CAD build for the part. Positions are in the model's coordinates, mm. Give positions to 0.01 mm unless a question says otherwise; leave off trailing zeros. Loops run counter-clockwise (first coordinate to the right, second up) from the corner with the lowest first, then second, coordinate; pieces in that order, holes last. Notation, with made-up numbers: M 67,46 L 90,46 A32 cw 90,76 Z; hole C -0.75,3 d5. An arc over 180 degrees is marked long. Answer as CSV lines item,"result".
```python
from build123d import *

# Parameters (mm, degrees)
ESQUISSE1_W             = 233
ESQUISSE1_H             = 150
BOSS_EXTRU_1_DEPTH      = 4.2
ESQUISSE2_R             = 2.55
ENL_V_MAT_EXTRU_1_DEPTH = 145.628460094


with BuildPart() as part:
    # Esquisse1 → Boss.-Extru.1 (new body)
    with BuildSketch(Plane.XY):
        with Locations((-3.063037439, -6.267653759)):
            Rectangle(ESQUISSE1_W, ESQUISSE1_H)
    extrude(amount=BOSS_EXTRU_1_DEPTH)

    # Esquisse2 → Enlèv. mat.-Extru.1 (cut, through all)
    with BuildSketch(Plane.XY.offset(4.2)):
        with Locations((-78.063037439, -47.267653759)):
            Circle(ESQUISSE2_R)
        with Locations((-1.063037439, -47.267653759)):
            Circle(ESQUISSE2_R)
        with BuildLine():
            Line((-69.563037439, -81.267653759), (-9.563037439, -81.267653759))
            ThreePointArc((-9.563037439, -81.267653759), (-39.563037439, -51.267653759), (-69.563037439, -81.267653759))
        make_face()
    extrude(amount=-ENL_V_MAT_EXTRU_1_DEPTH, mode=Mode.SUBTRACT)


solid = part.part
```
Q1. Cut at C-C (x = -61). Write the cut outline in (y, z), and give its area (3 significant figures).
Solution:
outline,"M -60.28,0 L 68.73,0 L 68.73,4.2 L -60.28,4.2 Z"
area,"542 mm²"
Q2. Wall check: line 1 (X direction, y = -45, z = 1.15); line 2 (X direction, y = -59, z = 1.7); line 3 (X direction, y = -64, z = 1.45). Give the ranges that are in metal, low to high. Write a range as [from, to].
Solution:
line 1,"x = [-119.56, -79.23], [-76.9, -2.23], [0.1, 113.44]"
line 2,"x = [-119.56, -59.67], [-19.46, 113.44]"
line 3,"x = [-119.56, -64.1], [-15.03, 113.44]"
Q3. Cut at A-A (y = -64.5). Write the cut outline in (x, z), and give its area (3 significant figures).
Solution:
outline,"M -119.56,0 L -64.44,0 L -64.44,4.2 L -119.56,4.2 Z; M -14.69,0 L 113.44,0 L 113.44,4.2 L -14.69,4.2 Z"
area,"770 mm²"
Q4. Cut at B-B (z = 2). Write the cut outline in (x, y).
Solution:
outline,"M -119.56,-81.27 L -69.56,-81.27 A30 cw -9.56,-81.27 L 113.44,-81.27 L 113.44,68.73 L -119.56,68.73 Z; hole C -78.06,-47.27 d5.1; hole C -1.06,-47.27 d5.1"
Q5. Mould opens along X. For faces 1 (the flat face through (51, -81.268, 2)), 2 (the flat face through (-119.563, -7, 2)), 3 (the cylindrical face through (-38.903, -51.275, 2.129)) say: released by +X, released by -X, zero draft, split by the parting line, or undercut.
Solution:
face 1,"zero draft"
face 2,"released by -X"
face 3,"undercut"
